Geometry: see drawing. Coordinates: mm, zero at the bounding-box minimum. Give positions to 0.01 mm unless a question says otherwise; leave off trailing zeros. Write each loop counter-clockwise with the first axis right and the second up, starting at its lowest first coordinate (ties: lowest second). Pieces come first, ordered by that corner, then holes. Notation, with made-up numbers: (-32, 89) -> (-5, 89) arc R6 ccw to (-5, 99) -> close; hole circle Ø1 at (60.25, 10). An arc over 180 degrees is marked (long way). Write item = value, one per line.
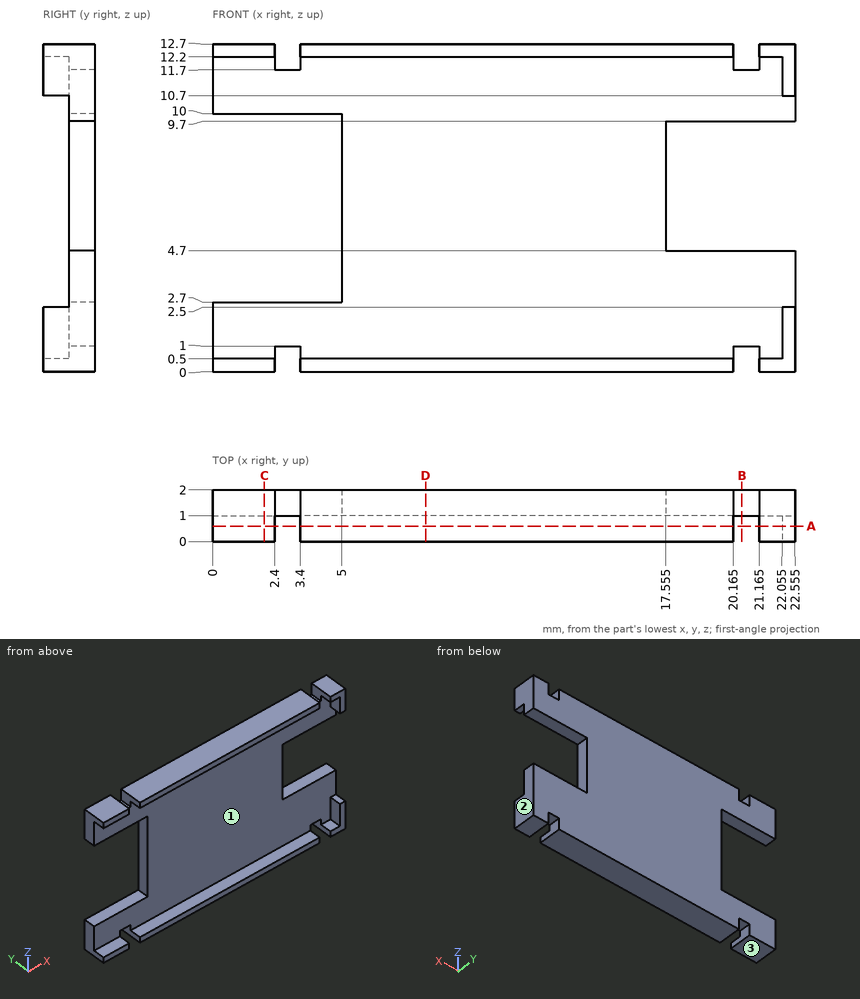
(1) First-contact query: pin 1 (0.8 mm diameter, centred on x = 19, y = 1.5, fed in from -Z); pin 2 (1 mm diameter, centred on y = 2, z = 7, fed in from +X) (3 decimals); pin 3 (4 mm diameter, centred on x = 7.5, z = 6, fed in from -Y); pin 4 (0.8 mm diameter, centred on y = 0.5, z = 1, fed in from -X) (3 decimals). Flat tips, straight axial feed; report the tip coordinate or a pass-through.
Values follow:
pin_1 = 0
pin_2 = 17.555
pin_3 = 1
pin_4 = 22.055
(2) Section query A-A (y = 0.6). Return loops of the section in (x, z) (1 decimal), plus the area to 3 significant figures.
Values follow:
outline = (0, 0) -> (2.4, 0) -> (2.4, 0.5) -> (0, 0.5) -> close; (0, 12.2) -> (2.4, 12.2) -> (2.4, 12.7) -> (0, 12.7) -> close; (3.4, 0) -> (20.2, 0) -> (20.2, 0.5) -> (3.4, 0.5) -> close; (3.4, 12.2) -> (20.2, 12.2) -> (20.2, 12.7) -> (3.4, 12.7) -> close; (21.2, 0) -> (22.6, 0) -> (22.6, 2.5) -> (22.1, 2.5) -> (22.1, 0.5) -> (21.2, 0.5) -> close; (21.2, 12.2) -> (22.1, 12.2) -> (22.1, 10.7) -> (22.6, 10.7) -> (22.6, 12.7) -> (21.2, 12.7) -> close
area = 22.3 mm2
(3) Pull-direction query (Z, two-part tool) for the marked faces 1, 2 and 3; classes: pulls with the +Z half, pulls with the -Z half, needs draft (parallel to the pull), parting line crosses it, or undercut.
Values follow:
face_1 = undercut
face_2 = needs draft
face_3 = pulls with the -Z half
(4) Material intervals for line 1 (X direction, y = 0.35, z = 12.25) (1 decimal); line 2 (Z direction, x = 3.25, y = 1.7); line 3 (Z direction, x = 9.5, y = 0.65), sorted ascending.
Values follow:
line_1 = 0 to 2.4, 3.4 to 20.2, 21.2 to 22.6
line_2 = 1 to 2.7, 10 to 11.7
line_3 = 0 to 0.5, 12.2 to 12.7
(5) Section query B-B (x = 20.5). Return loops of the section in (y, z).
Values follow:
outline = (1, 1) -> (2, 1) -> (2, 4.7) -> (1, 4.7) -> close; (1, 9.7) -> (2, 9.7) -> (2, 11.7) -> (1, 11.7) -> close
(6) Section query D-D (x = 8.25). Return loops of the section in (y, z).
Values follow:
outline = (0, 0) -> (2, 0) -> (2, 12.7) -> (0, 12.7) -> (0, 12.2) -> (1, 12.2) -> (1, 0.5) -> (0, 0.5) -> close
(7) Section query C-C (x = 2). Return loops of the section in (y, z).
Values follow:
outline = (0, 0) -> (2, 0) -> (2, 2.7) -> (1, 2.7) -> (1, 0.5) -> (0, 0.5) -> close; (0, 12.2) -> (1, 12.2) -> (1, 10) -> (2, 10) -> (2, 12.7) -> (0, 12.7) -> close
